The listing builds one solid part. Answer for the finished solid, in the listing's coordinates (mm). Round coordinates to 2 decimals unless told otherwise and drop trailing zeros. Write each loop counter-clockwise with the first axis right and the second up, starting at its lowest first coordinate (ties: lowest second). Pieces come first, ordered by that corner, then holes. Notation, with made-up numbers: (89, -29) - (131, -29) arc R12 cw to (131, -20) - close; hole circle Ø9 at (89.25, 22). An arc over 180 degrees is marked (long way). Answer as CSV lines item,"result". Start each with the question number.
Item 1: Straight lines are drawn through the part: line 1 along Z through (x, y) = (114, -0.1); line 2 along Z through (x, y) = (25, -0.2). For each, find the intervals that lie inside material, in ascending order. Write a range as [from, to].
Item 2: A cutting plane is placed at A-A on x = 25. Determine the outline of the cut face in (y, z), and give its area (3 significant figures).
Item 3: A cutting plane is placed at B-B on y = -0.2. State how many separate pieces and enclosed holes the cut face has, and give its area (3 significant figures).
```python
from build123d import *

# Parameters (mm, degrees)
SKETCH006_W   = 120.016
SKETCH006_H   = 20
SKETCH006_R   = 3.25
SKETCH006_R_2 = 3
SKETCH006_R_3 = 4.75
PAD_DEPTH     = 0.4


with BuildPart() as part:
    # Sketch006 → Pad (new body)
    with BuildSketch(Plane.XZ):
        with Locations((73.008, 14)):
            Rectangle(SKETCH006_W, SKETCH006_H)
        with Locations((25, 12.67)):
            Circle(SKETCH006_R, mode=Mode.SUBTRACT)
        with Locations((40.505, 13.9525)):
            Circle(SKETCH006_R_2, mode=Mode.SUBTRACT)
        with Locations((65.495, 13.9525)):
            Circle(SKETCH006_R_2, mode=Mode.SUBTRACT)
        with Locations((80.327, 14.17)):
            Circle(SKETCH006_R_3, mode=Mode.SUBTRACT)
        with Locations((96.026, 13.9525)):
            Circle(SKETCH006_R_2, mode=Mode.SUBTRACT)
        with Locations((121.016, 13.9525)):
            Circle(SKETCH006_R_2, mode=Mode.SUBTRACT)
        with BuildLine():
            Line((46.549023, 8.9525), (59.450977, 8.9525))
            ThreePointArc((59.450977, 8.9525), (60.479437, 9.326829), (61.026669, 10.274663))
            Line((62.225692, 17.074663), (61.026669, 10.274663))
            ThreePointArc((62.225692, 17.074663), (61.875671, 18.38096), (60.65, 18.9525))
            Line((60.65, 18.9525), (45.35, 18.9525))
            ThreePointArc((45.35, 18.9525), (44.124329, 18.38096), (43.774308, 17.074663))
            Line((43.774308, 17.074663), (44.973331, 10.274663))
            ThreePointArc((44.973331, 10.274663), (45.520563, 9.326829), (46.549023, 8.9525))
        make_face(mode=Mode.SUBTRACT)
        with BuildLine():
            Line((102.070023, 8.9525), (114.971977, 8.9525))
            ThreePointArc((114.971977, 8.9525), (116.000437, 9.326829), (116.547669, 10.274663))
            Line((117.746692, 17.074663), (116.547669, 10.274663))
            ThreePointArc((117.746692, 17.074663), (117.396671, 18.38096), (116.171, 18.9525))
            Line((116.171, 18.9525), (100.871, 18.9525))
            ThreePointArc((100.871, 18.9525), (99.645329, 18.38096), (99.295308, 17.074663))
            Line((99.295308, 17.074663), (100.494331, 10.274663))
            ThreePointArc((100.494331, 10.274663), (101.041563, 9.326829), (102.070023, 8.9525))
        make_face(mode=Mode.SUBTRACT)
    extrude(amount=PAD_DEPTH)


solid = part.part
```
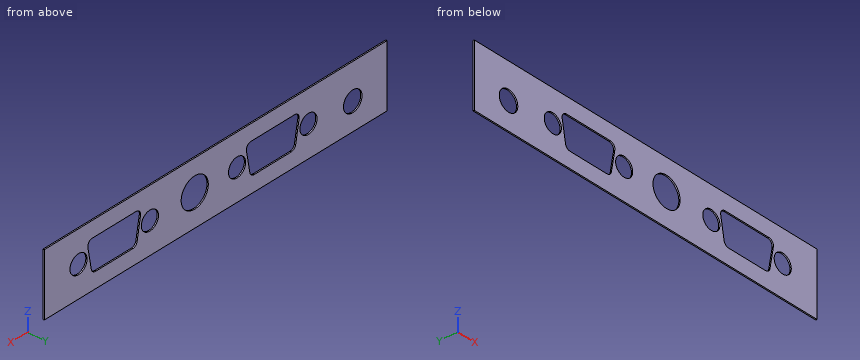
Geometry says:
1,line 1,"z = [4, 8.95], [18.95, 24]"
1,line 2,"z = [4, 9.42], [15.92, 24]"
2,outline,"(-0.4, 4) - (0, 4) - (0, 9.42) - (-0.4, 9.42) - close; (-0.4, 15.92) - (0, 15.92) - (0, 24) - (-0.4, 24) - close"
2,area,"5.40 mm^2"
3,separate pieces,"1"
3,enclosed holes,"8"
3,area,"1,840 mm^2"
